from build123d import *

# Parameters (mm, degrees)
SKETCH1_R           = 6
SKETCH1_R_2         = 3
BOSS_EXTRUDE1_DEPTH = 2
SKETCH2_R           = 5.5
SKETCH2_R_2         = 4
CUT_EXTRUDE1_DEPTH  = 0.2
FILLET1_R           = 0.4


with BuildPart() as part:
    # Sketch1 → Boss-Extrude1 (new body, symmetric)
    with BuildSketch(Plane.XY):
        Circle(SKETCH1_R)
        Circle(SKETCH1_R_2, mode=Mode.SUBTRACT)
    extrude(amount=BOSS_EXTRUDE1_DEPTH, both=True)

    # Sketch2 → Cut-Extrude1 (cut)
    with BuildSketch(Plane.XY.offset(2)):
        Circle(SKETCH2_R)
        Circle(SKETCH2_R_2, mode=Mode.SUBTRACT)
    cut_extrude1 = extrude(amount=-CUT_EXTRUDE1_DEPTH, mode=Mode.SUBTRACT)

    # Mirror1: Cut-Extrude1 across plane
    add(cut_extrude1.mirror(Plane.XY), mode=Mode.SUBTRACT)

    # Fillet1
    fillet1_edges = [part.edges().sort_by_distance(p)[0] for p in [
        (-6, 0, -2),
        (-6, 0, 2),
        (-3, 0, -2),
        (-3, 0, 2),
    ]]
    fillet(fillet1_edges, radius=FILLET1_R)


solid = part.part
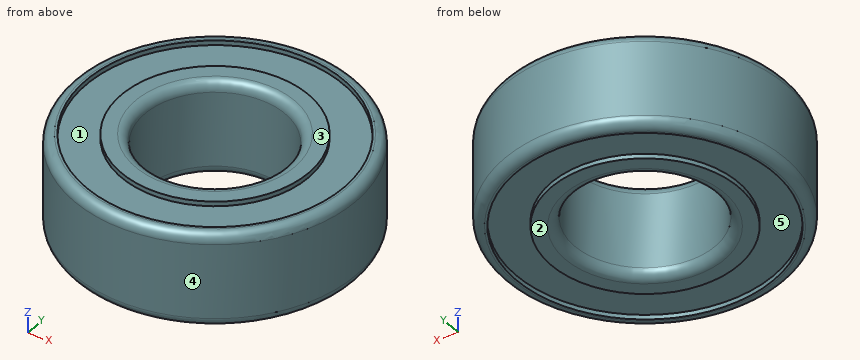
Read the model definition and answer for the solid it produces. Units are mm, in the model's axes. Face numbers are marked on the shaded views. A direction names the side the tool comes from. Give positions to 0.01 mm unless a question says otherwise; leave off trailing zeros. Write each loop counter-clockwise with the first axis right and the second up, starting at its lowest first coordinate (ties: lowest second). Pieces come first, ordered by that corner, then holes. Notation, with made-up numbers: M -38.5,38 L -6.5,38 A17 cw -6.5,63 Z; hole C 35,-34.75 d5. An arc over 180 degrees is marked long. One line per item, written item: value. Start each with the question number.
(1) A tool of negligible diameter and unlimited length cuts with its end or side. For the marked faces 1 and 2, from which of +Z, -Z, +X, -X, +Y, -Y can it reach the whole face along a straight path? Write none if from no direction.
(2) Find section C-C (z = 0.95). Determine the outline of the cut face in (x, y).
(3) Flat-ended cylindrical pins translate along their axes: pin 1 Ø1.5 at (x, y) = (4, 3) entering from +Z; pin 2 Ø2 at (y, z) = (-4.5, 0) entering from -X; pin 3 Ø3.5 at (x, y) = (-1, -1) entering from -Z. Find the tip coordinate at first contact, or state that the pin passes through.
(4) Determine the mould class of the marked faces 3, 4 and 5 for opening direction Y: pulls with the +Y half, pulls with the -Y half, needs draft (parallel to the pull), parting line crosses it, or undercut.
(5) Find the intervals of material crossed by line 1 (Y direction, x = 0, z = -0.25); line 2 (Y direction, x = 0, z = 1.9); line 3 (Z direction, x = 4.5, y = 1), in increasing order.
Results below:
1. face 1: +Z
1. face 2: -Z, +X, -X, +Y, -Y
2. outline: C 0,0 d12; hole C 0,0 d6
3. pin 1: stops at z = 2
3. pin 2: stops at x = -4.87
3. pin 3: stops at z = -1.92
4. face 3: needs draft
4. face 4: parting line crosses it
4. face 5: undercut
5. line 1: y = -6 to -3, 3 to 6
5. line 2: y = -5.86 to -5.5, -4 to -3.14, 3.14 to 4, 5.5 to 5.86
5. line 3: z = -1.8 to 1.8
